Design review of the part built by this model. Coordinates are the model's own, in mm. Face numbers are marked on the shaded views. A direction names the side the tool comes from. Coordinates: 2 decimals unless noted, no trailing zeros. Order: outer loops, then holes, each group sorted by start corner. A loop starts at its lowest first (then second) coordinate and runs counter-clockwise, first axis right, second up. Notation, with made-up numbers: M 23,10.25 L 27,10.25 A26 ccw 27,40.25 Z; hole C -33,49 d2. An arc over 180 degrees is marked long. Answer in a Markdown table with one row per item.
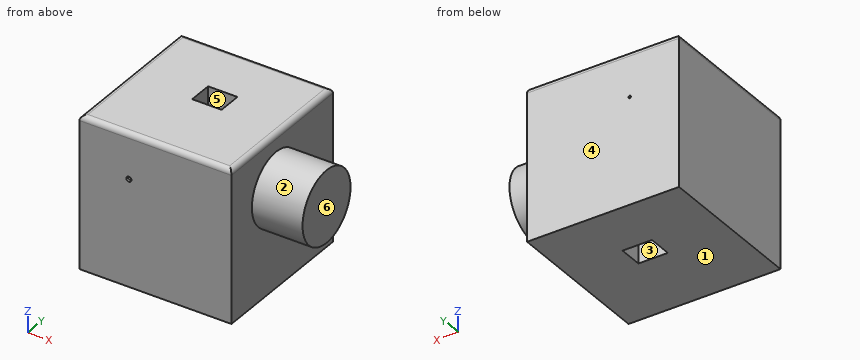
from build123d import *

# Parameters (mm, degrees)
F0_W           = 381
F0_H           = 381
F1_DEPTH       = 381
F3_D           = 6.35
F3_CSINK_D     = 12.7
F3_CSINK_ANGLE = 90
F4_R           = 12.7
F5_R           = 90.072303
F6_DEPTH       = 127
F7_W           = 73.772475
F7_H           = 59.68143
F8_DEPTH       = 508


with BuildPart() as f1:
    # F0 (on Front) → F1 (new body)
    with BuildSketch(Plane.XZ):
        with Locations((190.5, 190.5)):
            Rectangle(F0_W, F0_H)
    extrude(amount=F1_DEPTH)

    # F3 (through all)
    with Locations(Plane.XZ.offset(381)):
        with Locations((123.825006, 267.081022)):
            CounterSinkHole(F3_D / 2, F3_CSINK_D / 2, counter_sink_angle=F3_CSINK_ANGLE)

    # F4
    f4_edges = [f1.edges().sort_by_distance(p)[0] for p in [
        (381, -190.5, 381),
        (0, -190.5, 381),
        (190.5, 0, 381),
        (190.5, -381, 381),
    ]]
    fillet(f4_edges, radius=F4_R)

    # F5 (on face) → F6 (join)
    with BuildSketch(Plane.YZ.offset(381)):
        with Locations((-214.303002, 247.298166)):
            Circle(F5_R)
    extrude(amount=F6_DEPTH)

    # F7 (on face) → F8 (cut)
    with BuildSketch(Plane.XY.offset(381)):
        with Locations((197.570882, -168.751098)):
            Rectangle(F7_W, F7_H)
    extrude(amount=-F8_DEPTH, mode=Mode.SUBTRACT)


solid = f1.part
(1) For the marked faces 1, 2 and 3, list the 3-axis set-ups (+Z, -Z, +X, -X, +Y, -Y) from which the entire face can be reached by the end or side of a thin tool; tool diameter is ignored.
Return value:
| item | result |
|---|---|
| face 1 | -Z, +X, -X, +Y, -Y |
| face 2 | +X |
| face 3 | +Z, -Z |
(2) Add section B-B, the plane y = -167. Give the boundary of the cut face in (x, z) (3 decimals), and give its area (3 significant figures).
Return value:
| item | result |
|---|---|
| outline | M 0,0 L 160.685,0 L 160.685,381 L 12.7,381 A12.7 ccw 0,368.3 Z; M 234.457,0 L 381,0 L 381,170.647 L 508,170.647 L 508,323.95 L 381,323.95 L 381,368.3 A12.7 ccw 368.3,381 L 234.457,381 Z; hole C 123.825,267.081 d6.35 |
| area | 136,000 mm2 |
(3) Add section C-C, the plane x = 179.5. Give the boundary of the cut face in (y, z), and give its area (3 significant figures).
Return value:
| item | result |
|---|---|
| outline | M -381,0 L -198.59,0 L -198.59,381 L -368.3,381 A12.7 ccw -381,368.3 Z; M -138.91,0 L 0,0 L 0,368.3 A12.7 ccw -12.7,381 L -138.91,381 Z |
| area | 122,000 mm2 |
(4) Insertion check: pin 1 Ø4 at (y, z) = (-160, 71.5) entering from +X; pin 2 Ø2 at (x, y) = (421.5, -133.5) entering from +Z; pin 3 Ø5 at (x, z) = (123.83, 267.08) entering from -Y. Each pin has a flat end and moves straight along its axis. Give the tip position at first contact, or say it passes through.
Return value:
| item | result |
|---|---|
| pin 1 | stops at x = 381 |
| pin 2 | stops at z = 289.07 |
| pin 3 | passes through |
(5) Add section A-A, the plane z = 97.5. Give the boundary of the cut face in (x, y), and give its area (3 significant figures).
Return value:
| item | result |
|---|---|
| outline | M 0,-381 L 381,-381 L 381,0 L 0,0 Z; hole M 160.68,-198.59 L 234.46,-198.59 L 234.46,-138.91 L 160.68,-138.91 Z |
| area | 141,000 mm2 |
(6) Draft analysis for pull direction Y (two halves, no side actions). For the marked faces 4, 5 and 6, state which applies: pulls with the +Y half, pulls with the -Y half, needs draft (parallel to the pull), parting line crosses it, or undercut.
Return value:
| item | result |
|---|---|
| face 4 | pulls with the +Y half |
| face 5 | undercut |
| face 6 | needs draft |
(7) Add section D-D, the plane y = -275.5. Give the boundary of the cut face in (x, z) (3 decimals), and give its area (3 significant figures).
Return value:
| item | result |
|---|---|
| outline | M 0,0 L 381,0 L 381,181.208 L 508,181.208 L 508,313.389 L 381,313.389 L 381,368.3 A12.7 ccw 368.3,381 L 12.7,381 A12.7 ccw 0,368.3 Z; hole C 123.825,267.081 d6.35 |
| area | 162,000 mm2 |
(8) For line 1 along Y through (x, z) = (219.5, 114.5); line 2 along X through (y, z) = (-95.5, 25.5); line 3 along Y through (x, z) = (471, 300.5), list the stretches that pass through material, from the lowest coordinate up. Write a range as from..to.
Return value:
| item | result |
|---|---|
| line 1 | y = -381..-198.59, -138.91..0 |
| line 2 | x = 0..381 |
| line 3 | y = -286.98..-141.62 |
